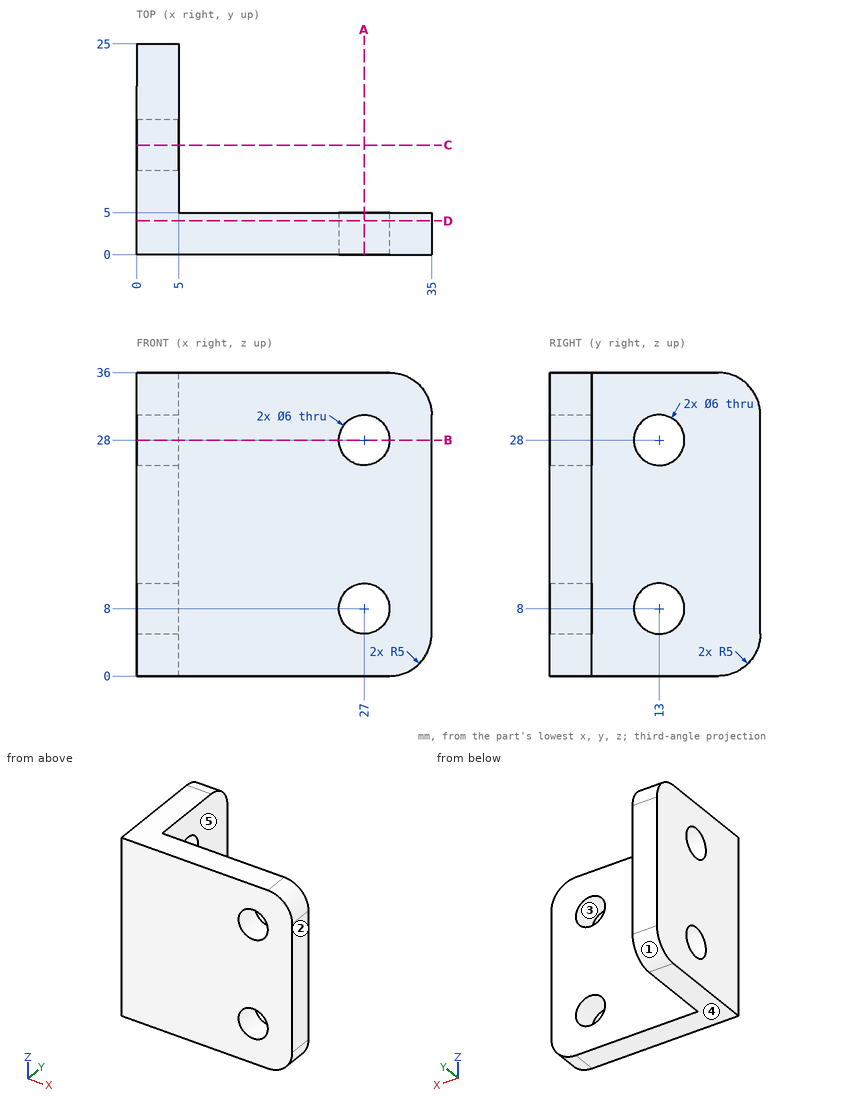
Can you work these out from the drawing? Everything is in mm from the part's minimum corner. A direction names the side the tool comes from. Give positions to 0.01 mm unless a question says otherwise; leave off trailing zeros. Order: outer loops, then holes, each group sorted by start corner. A loop starts at its lowest first (then second) coordinate and runs counter-clockwise, first axis right, second up.
1. For the marked faces 4 and 5, which set-ups out of +Z, -Z, +X, -X, +Y, -Y let a thin tool reach every point of the face, with its end or its side?
2. Suppose I cut it at B-B (z = 28). List the corners of the cut face in (x, y) for me, plus the area to 3 significant figures.
3. We'd pull the mould along X, two halves only. Please class the marked faces 1, 2 and 3: pulls with the +X half, pulls with the -X half, needs draft (parallel to the pull), parting line crosses it, or undercut.
4. Will these pins go through, and if not, where does the flat tip stop? P1, Ø5.5, axis at x = 27, z = 28, coming from the +Y side; P2, Ø5, axis at x = 20, z = 10, coming from the +Y side.
5. Suppose I cut it at D-D (y = 4). List the corners of the cut face in (x, z) for me.
6. I need wall thicknesses on L1, parallel to Z at x = 27, y = 3.5; L2, parallel to Y at x = 20, z = 32. Which ranges of each line are inside material? Lowest first, please.
7. Suppose I cut it at A-A (x = 27). List the corners of the cut face in (y, z) for me.
Solved:
1. face 4: -Z, +X, -X, +Y, -Y
1. face 5: +Z, -Z, +X, +Y
2. outline: (0, 0) - (24, 0) - (24, 5) - (5, 5) - (5, 10) - (0, 10) - close; (0, 16) - (5, 16) - (5, 25) - (0, 25) - close; (30, 0) - (35, 0) - (35, 5) - (30, 5) - close
2. area: 215 mm2
3. face 1: needs draft
3. face 2: pulls with the +X half
3. face 3: undercut
4. P1: passes through
4. P2: stops at y = 5
5. outline: (0, 0) - (30, 0) arc R5 ccw to (35, 5) - (35, 31) arc R5 ccw to (30, 36) - (0, 36) - close; hole circle Ø6 at (27, 8); hole circle Ø6 at (27, 28)
6. L1: z = 0 to 5, 11 to 25, 31 to 36
6. L2: y = 0 to 5
7. outline: (0, 0) - (5, 0) - (5, 5) - (0, 5) - close; (0, 11) - (5, 11) - (5, 25) - (0, 25) - close; (0, 31) - (5, 31) - (5, 36) - (0, 36) - close
